Could you check a few things on this model? Use its own coordinates, in mm. Face numbers are marked on the shaded views. A direction names the side the tool comes from. Coordinates: 2 decimals unless noted, no trailing zeros. Order: outer loops, then holes, each group sorted by start corner. A loop starts at its lowest first (then second) coordinate and runs counter-clockwise, first axis right, second up. Notation, with made-up numbers: (38, 11) - (43, 11) arc R28 ccw to (43, 49) - close; hole circle Ø5 at (52.5, -33). An arc over 180 degrees is marked (long way). Answer as a JSON object with one key per item and string values. Group by question number.
(1) Imagine slicing it at D-D, the plane y = -3.5. Write out the boundary of the cut face in (x, z), and give its area (3 significant figures).
(2) Which directions (+Z, -Z, +X, -X, +Y, -Y) give clear straight access to the entire face, cutting with the end or side of a thin tool? Please do the marked faces 4, 5 and 6.
(3) Will these pins go through, and if not, where does the flat tip stop? P1, Ø3, axis at x = -0.5, z = -1, coming from the -Y side; P2, Ø4, axis at x = -1.5, y = 8.5, coming from the -Z side.
(4) We'd pull the mould along Z, two halves only. Please class the marked faces 1, 2 and 3: pulls with the +Z half, pulls with the -Z half, needs draft (parallel to the pull), parting line crosses it, or undercut.
(5) Please list where these lines run through material, in increasing order: probe 1 along X at (y, z) = (7.75, 2.2); probe 2 along Z at (x, y) = (4.5, 9); probe 3 along Z at (x, y) = (3.75, 8.25).
(6) Imagine slicing it at B-B, the plane y = 7.5. Write out the boundary of the cut face in (x, z), and give its area (3 significant figures).
(7) Imagine slicing it at A-A, the plane z = 0. Write out the boundary of the cut face in (x, y).
(8) Imagine slicing it at C-C, the plane x = 0. Write out the boundary of the cut face in (y, z), and give its area (3 significant figures).
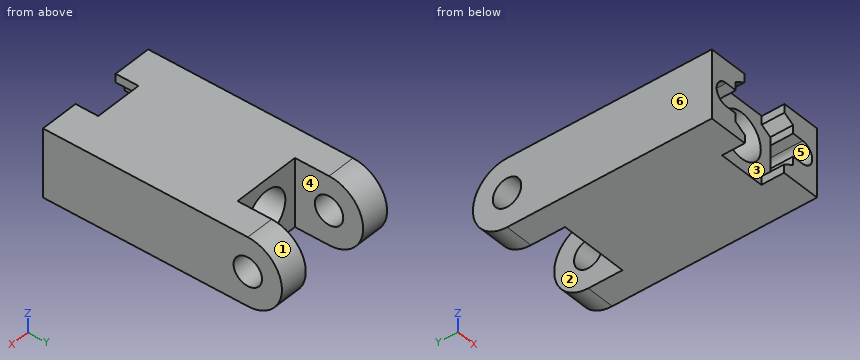
Autodesk Inventor part; units mm, degrees
ref_plane "plane_support" through (-5.5, -8, -3) normal (0, -1, 0) x (1, 0, 0)
ref_plane "plane_support_frontb" through (-2.5, 0, 0) normal (1, 0, 0) x (0, 0, -1)
ref_plane "plane_support_frontt" through (2.5, 0, 0) normal (-1, 0, 0) x (0, 0, 1)
sketch "Sketch14" plane through (0, 0, 0) normal (1, 0, 0) x (0, 1, 0)
  line L0 (-13.2, 0) -> (16.2, 0)
  line L1 (0, -4.2) -> (0, 4.2)
  line L2 (9, -3) -> (-9, -3)
  line L3 (-9, -3) -> (-9, 3)
  line L4 (-9, 3) -> (9, 3)
  line L5 (9, 3) -> (9, -3) construction
  line L6 (9, -3) -> (-9, 3) construction
  line L7 (-9, -3) -> (9, 3) construction
  line L8 (5.5, 3) -> (5.5, -3) construction
  line L9 (-6.5, 3) -> (-6.5, -3) construction
  arc A0 (9, -3) -> (9, 3) centre (9, 0) ccw
  circle A1 centre (9, 0) radius 1.25
  circle A2 centre (9, 0) radius 3 construction
  line L10 (6, 3) -> (6, -3) construction
  point P0 (0, 0)
  point P1 (0, 0)
  dimension "d72" = 6
  dimension "d73" = 12
  dimension "d74" = 2.5
  dimension "d75" = 2.5
  dimension "d76" = 0.5
extrude "ext_main" add sketch "Sketch14" along normal mid plane 11 contours L3 L4 L1 L0 | L0 L1 L2 L3 | L1 L4 A0 L0 A1 | L0 A1 A0 L2 L1
sketch "Sketch15" plane through (0, 0, 0) normal (1, 0, 0) x (0, 1, 0)
  circle A0 centre (9, 0) radius 1.25
  arc A1 (9, -3) -> (9, 3) centre (9, 0) ccw
  circle A2 centre (9, 0) radius 3
  line L0 (6, 3) -> (6, -3)
  line L1 (9, 3) -> (-9, 3)
  line L2 (-9, -3) -> (9, -3)
  line L3 (-13.2, 0) -> (16.2, 0)
  point P0 (0, 0)
extrude "ext_cut_front" cut sketch "Sketch15" along normal mid plane 6 contours L3 A1 A2 A0 | A0 L3 A2 A1 | L0 L1 A2 | A2 L2 L0
sketch "sk_channel_nut" plane through (-5.5, -9, -3) normal (0, -1, 0) x (1, 0, 0)
  line L0 (-2.2, 3) -> (13.2, 3)
  line L1 (5.5, -1.8497) -> (5.5, 7.8497)
  circle A0 centre (5.5, 3) radius 2
  line L2 (5.5, 6.4641) -> (2.5, 4.7321)
  line L3 (2.5, 4.7321) -> (2.5, 1.2679)
  line L4 (2.5, 1.2679) -> (5.5, -0.4641)
  line L5 (5.5, -0.4641) -> (8.5, 1.2679)
  line L6 (8.5, 1.2679) -> (8.5, 4.7321)
  line L7 (8.5, 4.7321) -> (5.5, 6.4641)
  circle A1 centre (1.5, 3) radius 1
  circle A2 centre (9.5, 3) radius 1
  line L8 (1.5, 4) -> (2.5, 4)
  line L9 (1.5, 2) -> (2.5, 2)
  line L10 (9.5, 4) -> (8.5, 4)
  line L11 (9.5, 2) -> (8.5, 2)
  line L12 (11, 0) -> (0, 0)
  line L13 (11, 6) -> (0, 6)
  line L14 (0, 0) -> (0, 6)
  line L15 (3.4, 6) -> (3.4, 5.2517)
  line L16 (3.4456, 0.722) -> (3.4456, 0)
  line L17 (7.5544, 0.722) -> (7.5544, 0)
  line L18 (7.6, 6) -> (7.6, 5.2517)
  point P0 (5.5, 3)
  point P1 (2.5, 3)
  dimension "d85" = 4
  dimension "d86" = 120
  dimension "d87" = 6
  dimension "d88" = 2
  dimension "d95" = 4.2
extrude "ext_cut_channel" cut sketch "sk_channel_nut" against normal up to surface (15 mm away) contours A0 L1 L0 | L0 L1 A0 | L1 A0 L0 | L0 A0 L1
extrude "ext_cut_bottomscrews" cut sketch "sk_channel_nut" against normal blind 8 contours A1 L0 | L0 A1 | A1 L8 L3 | L3 L9 A1 | A2 L0 | A2 L11 L6 | L6 L10 A2 | L0 A2
extrude "ext_cut_bottom_nut" cut sketch "sk_channel_nut" against normal blind 2 contours L3 L2 L13 L1 A0 L0 | L0 A0 L1 L12 L4 L3 | L16 L4 L12 | L13 L2 L15 | A0 L1 L0 | L0 L1 A0 | L12 L1 L4 | L2 L1 L13 | L1 A0 L0 | L0 A0 L1 | L1 L13 L7 L6 L0 A0 | A0 L0 L6 L5 L12 L1 | L1 L12 L5 | L7 L13 L1 | L5 L17 L12 | L13 L18 L7
sketch "Sketch19" plane through (-5.5, -8, -3) normal (0, -1, 0) x (1, 0, 0)
  line L0 (3.4, 6) -> (7.6, 6)
  line L1 (3.4, 5.2517) -> (3.4, 6)
  line L2 (2.5, 4.7321) -> (3.4, 5.2517)
  line L3 (2.5, 4) -> (2.5, 4.7321)
  line L4 (2.5, 2) -> (2.5, 4)
  line L5 (2.5, 1.2679) -> (2.5, 2)
  line L6 (3.4456, 0.722) -> (2.5, 1.2679)
  line L7 (3.4456, 0) -> (3.4456, 0.722)
  line L8 (7.5544, 0) -> (3.4456, 0)
  line L9 (7.5544, 0.722) -> (7.5544, 0)
  line L10 (8.5, 1.2679) -> (7.5544, 0.722)
  line L11 (8.5, 2) -> (8.5, 1.2679)
  line L12 (8.5, 4) -> (8.5, 2)
  line L13 (8.5, 4.7321) -> (8.5, 4)
  line L14 (7.6, 5.2517) -> (8.5, 4.7321)
  line L15 (7.6, 6) -> (7.6, 5.2517)
  circle A0 centre (5.5, 3) radius 2
  line L16 (3.9, 5.5) -> (7.1, 5.5) construction
  line L17 (7.1, 5.5) -> (7.1, 4.963)
  line L18 (7.1, 4.963) -> (8, 4.4434)
  line L19 (8, 4.4434) -> (8, 4)
  line L20 (8, 4) -> (8, 2)
  line L21 (8, 2) -> (8, 1.5566)
  line L22 (8, 1.5566) -> (7.0544, 1.0107)
  line L23 (7.0544, 1.0107) -> (7.0544, 0.5)
  line L24 (7.0544, 0.5) -> (3.9456, 0.5) construction
  line L25 (3.9456, 0.5) -> (3.9456, 1.0107)
  line L26 (3.9456, 1.0107) -> (3, 1.5566)
  line L27 (3, 1.5566) -> (3, 2)
  line L28 (3, 2) -> (3, 4)
  line L29 (3, 4) -> (3, 4.4434)
  line L30 (3, 4.4434) -> (3.9, 4.963)
  line L31 (3.9, 4.963) -> (3.9, 5.5)
  line L32 (3.9, 5.5) -> (7.1, 5.5)
  line L33 (7.1, 5.5) -> (7.1, 6)
  line L34 (7.1, 6) -> (3.9, 6)
  line L35 (3.9, 6) -> (3.9, 5.5)
  line L36 (3.9456, 0.5) -> (7.0544, 0.5)
  line L37 (7.0544, 0.5) -> (7.0544, 0)
  line L38 (7.0544, 0) -> (3.9456, 0)
  line L39 (3.9456, 0) -> (3.9456, 0.5)
  point P0 (5.5, 3)
  dimension "d97" = 0.4
sketch "Sketch20" plane through (-2.5, 0, 0) normal (1, 0, 0) x (0, 0, -1)
  circle A0 centre (0, 9) radius 1.25
  arc A1 (3, 9) -> (-3, 9) centre (0, 9) ccw
  line L0 (-3, 6) -> (-3, 9)
  line L1 (3, 6) -> (-3, 6)
  line L2 (3, 9) -> (3, 6)
  line L3 (-3, 7) -> (3, 7)
  point P0 (0, 0)
  dimension "d102" = 1
equation "\"d73\" = linact_rod_effective_length"
equation "\"d74\" = nut_m3_thickness_max"
equation "\"d75\" = screw_m2_bore_loose"
equation "\"d87\" = nut_m3_width_acrossflats"
equation "\"d88\" = screw_m2_bore_selfthreading"
equation "\"d95\" = 0.7 * nut_m3_width_acrossflats"
equation "\"d89\" = linact_rod_effective_length + nut_m3_thickness_max"
equation "\"d93\" = 0.8 * nut_m3_thickness_max"
equation "\"d97\" = print_support_z_clearance"
equation "\"d102\" = print_support_xy_clearance"
equation "\"d96\" = print_support_xy_clearance"
equation "\"d100\" = print_support_z_clearance"
equation "\"d101\" = print_support_z_clearance"
properties part number "empty"
Result set:
{
 "1": {"outline": "(-5.5, -3) - (5.5, -3) - (5.5, 3) - (-5.5, 3) - close; hole (-4, -1) - (-3, -1) - (-3, 1) - (-4, 1) arc R1 ccw to start; hole circle Ø4 at (0, 0); hole (3, -1) - (4, -1) arc R1 ccw to (4, 1) - (3, 1) - close", "area": "46.3 mm^2"},
 "2": {"face 4": "+Z, -Z, +Y", "face 5": "-Y", "face 6": "+Z, -Z, -X, +Y, -Y"},
 "3": {"P1": "stops at y = -7", "P2": "stops at z = -3"},
 "4": {"face 1": "parting line crosses it", "face 2": "needs draft", "face 3": "undercut"},
 "5": {"probe 1": "x = -5.5 to -3, 3 to 5.5", "probe 2": "z = -3 to -1.25, 1.25 to 3", "probe 3": "z = -3 to -1, 1 to 3"},
 "6": {"outline": "(-5.5, -3) - (-3, -3) - (-3, 3) - (-5.5, 3) - close; (3, -3) - (5.5, -3) - (5.5, 3) - (3, 3) - close", "area": "30.0 mm^2"},
 "7": {"outline": "(-5.5, -9) - (-5, -9) - (-5, -1) - (-3, -1) - (-3, -7) - (-2, -7) - (-2, 6) - (-3, 6) - (-3, 7.75) - (-5.5, 7.75) - close; (-5.5, 10.25) - (-3, 10.25) - (-3, 12) - (-5.5, 12) - close; (2, -7) - (3, -7) - (3, -1) - (5, -1) - (5, -9) - (5.5, -9) - (5.5, 7.75) - (3, 7.75) - (3, 6) - (2, 6) - close; (3, 10.25) - (5.5, 10.25) - (5.5, 12) - (3, 12) - close"},
 "8": {"outline": "(-7, -3) - (6, -3) - (6, -2) - (-7, -2) - close; (-7, 2) - (6, 2) - (6, 3) - (-7, 3) - close", "area": "26.0 mm^2"}
}
